Here's how the part is built. I have some questions about the finished solid (model axes, mm). A direction names the side the tool comes from. Round coordinates to 2 decimals unless told otherwise and drop trailing zeros. Write each loop counter-clockwise with the first axis right and the second up, starting at its lowest first coordinate (ties: lowest second). Pieces come first, ordered by that corner, then holes. Notation, with made-up numbers: (-16, 63) -> (-2, 63) arc R20 ccw to (-2, 92) -> close; hole circle Ø4 at (10.5, 26.25). An arc over 180 degrees is marked (long way). Answer as CSV lines item,"result".
Autodesk Inventor part; units mm, degrees
ref_plane "YZ Plane" through (0, 0, 0) normal (1, 0, 0) x (0, 1, 0)
ref_plane "XZ Plane" through (0, 0, 0) normal (0, 1, 0) x (-1, 0, 0)
ref_plane "XY Plane" through (0, 0, 0) normal (0, 0, 1) x (1, 0, 0)
sketch "Sketch1" plane through (0, 0, 0) normal (0, 1, 0) x (-1, 0, 0)
  line L0 (0, 0) -> (-25.4, 0)
  line L1 (-25.4, 0) -> (-25.4, -38.1)
  line L2 (-25.4, -38.1) -> (0, -38.1)
  line L3 (0, -38.1) -> (0, 0)
  dimension "d0" = 25.4
  dimension "d1" = 38.1
extrude "Extrusion1" add sketch "Sketch1" along normal blind 2.54
sketch "Sketch3" plane through (0, 2.54, 0) normal (0, 1, 0) x (1, 0, 0)
  line L0 (0, 0) -> (5.08, 0)
  line L1 (5.08, 0) -> (5.08, 4.064)
  line L2 (5.08, 4.064) -> (0, 4.064)
  line L3 (0, 4.064) -> (0, 0)
  line L4 (25.4, 38.1) -> (0, 38.1)
  line L5 (0, 38.1) -> (5.08, 38.1)
  line L6 (5.08, 38.1) -> (5.08, 34.036)
  line L7 (5.08, 34.036) -> (0, 34.036)
  line L8 (0, 34.036) -> (0, 38.1)
  line L9 (5.08, 4.064) -> (16.256, 4.064)
  line L10 (16.256, 4.064) -> (16.256, 34.036)
  line L11 (16.256, 34.036) -> (5.08, 34.036)
  line L12 (5.08, 34.036) -> (5.08, 4.064)
  dimension "d7" = 5.08
  dimension "d8" = 4.064
  dimension "d9" = 5.08
  dimension "d10" = 4.064
  dimension "d11" = 11.176
extrude "Extrusion2" cut sketch "Sketch3" against normal blind 2.54 contours L12 L11 L10 L9
sketch "Sketch4" plane through (0, 2.54, 0) normal (0, 1, 0) x (1, 0, 0)
  line L0 (25.4, 0) -> (25.4, 38.1)
  line L1 (25.4, 0) -> (22.86, 0)
  line L2 (22.86, 0) -> (22.86, 10.16)
  line L3 (22.86, 10.16) -> (25.4, 10.16)
  line L4 (25.4, 10.16) -> (25.4, 0)
  line L5 (25.4, 38.1) -> (22.86, 38.1)
  line L6 (22.86, 38.1) -> (22.86, 27.94)
  line L7 (22.86, 27.94) -> (25.4, 27.94)
  line L8 (25.4, 27.94) -> (25.4, 38.1)
  point P0 (0, 0)
  dimension "d14" = 2.54
  dimension "d15" = 10.16
  dimension "d16" = 2.54
  dimension "d17" = 10.16
extrude "Extrusion3" add sketch "Sketch4" along normal blind 20.32
sketch "Sketch5" plane through (22.86, 2.54, -10.16) normal (-1, 0, 0) x (0, 0, 1)
  line L0 (10.16, 20.32) -> (0, 20.32)
  line L1 (5.08, 20.32) -> (5.08, 10.16)
  point P0 (10.16, -2.54)
  dimension "d20" = 10.16
hole "Hole1" at (22.86, 12.7, -5.08) direction (1, 0, 0) diameter 5.08 end through all
sketch "Sketch6" plane through (22.86, 2.54, -38.1) normal (-1, 0, 0) x (0, 0, 1)
  line L0 (10.16, 20.32) -> (0, 20.32)
  line L1 (5.08, 20.32) -> (5.08, 10.16)
  point P0 (38.1, -2.54)
  dimension "d28" = 10.16
hole "Hole2" at (22.86, 12.7, -33.02) direction (1, 0, 0) diameter 5.08 end through all
fillet "Fillet1" radius 5.08 4 edges at (22.86, 2.54, -5.08) (22.86, 2.54, -33.02) (24.13, 2.54, -27.94) (24.13, 2.54, -10.16)
properties part number "Actobotics Power Switch Mount v2"
1. Suppose I cut it at B-B on y = 18.25. Please give me the cut outline in (x, z), and give its area (3 significant figures).
Numbers:
outline,"(22.86, -38.1) -> (25.4, -38.1) -> (25.4, -27.94) -> (22.86, -27.94) -> close; (22.86, -10.16) -> (25.4, -10.16) -> (25.4, 0) -> (22.86, 0) -> close"
area,"51.6 mm^2"
2. If we mould it in two halves opening along X, with no side actions, what happens to faces 1 (the face through (25.4, 1, -19)), 2 (the face through (24.15, 15.18, -5.63)), 3 (the face through (16.256, 1, -19))? For each: released by +X, released by -X, zero draft, split by the parting line, or undercut.
Numbers:
face 1,"released by +X"
face 2,"zero draft"
face 3,"undercut"
3. If I drill on line 1 (Z direction, x = 24.45, y = 12.7); line 2 (Y direction, x = 24.5, z = -5.08); line 3 (Z direction, x = 23.75, y = 18.5), over which ranges is the centre line in solid material (lowest first)?
Numbers:
line 1,"z = -38.1 to -35.56, -30.48 to -27.94, -10.16 to -7.62, -2.54 to 0"
line 2,"y = 0 to 10.16, 15.24 to 22.86"
line 3,"z = -38.1 to -27.94, -10.16 to 0"
4. On a 3-axis mill with a long thin cutter (end or side, diameter ignored), from which of +Z, -Z, +X, -X, +Y, -Y can I reach the whole of each face in a straight line? I mean faces 4 (the face through (11, 1, -4.064)), 5 (the face through (22.86, 15.13, -3.88)), 6 (the face through (24, 15, -10.16)). Say none if no direction works.
Numbers:
face 4,"+Y, -Y"
face 5,"+Z, -Z, -X, +Y"
face 6,"+X, -X, +Y"
5. Suppose I cut it at A-A on x = 12.5. Please give me the cut outline in (y, z).
Numbers:
outline,"(0, -38.1) -> (2.54, -38.1) -> (2.54, -34.04) -> (0, -34.04) -> close; (0, -4.06) -> (2.54, -4.06) -> (2.54, 0) -> (0, 0) -> close"
6. Suppose I cut it at D-D on z = -5.08. Please give me the cut outline in (x, y).
Numbers:
outline,"(0, 0) -> (5.08, 0) -> (5.08, 2.54) -> (0, 2.54) -> close; (16.26, 0) -> (25.4, 0) -> (25.4, 10.16) -> (22.86, 10.16) -> (22.86, 7.62) arc R5.08 cw to (17.78, 2.54) -> (16.26, 2.54) -> close; (22.86, 15.24) -> (25.4, 15.24) -> (25.4, 22.86) -> (22.86, 22.86) -> close"
7. For pin 1 Ø11 at (y, z) = (16, -7) entering from -X; pin 2 Ø8 at (y, z) = (10, -27.5) entering from -X, each with a flat end and sliding along its axis, tell me the tip position at first contact or that it passes through.
Numbers:
pin 1,"stops at x = 22.86"
pin 2,"stops at x = 22.6"
8. Suppose I cut it at C-C on y = 12.7. Please give me the cut outline in (x, z), and give its area (3 significant figures).
Numbers:
outline,"(22.86, -38.1) -> (25.4, -38.1) -> (25.4, -35.56) -> (22.86, -35.56) -> close; (22.86, -30.48) -> (25.4, -30.48) -> (25.4, -27.94) -> (22.86, -27.94) -> close; (22.86, -10.16) -> (25.4, -10.16) -> (25.4, -7.62) -> (22.86, -7.62) -> close; (22.86, -2.54) -> (25.4, -2.54) -> (25.4, 0) -> (22.86, 0) -> close"
area,"25.8 mm^2"
